Build history of the part. All positions in model axes, mm. Face numbers are marked on the shaded views. A direction names the side the tool comes from. Give positions to 0.01 mm unless a question says otherwise; leave off trailing zeros. Write each loop counter-clockwise with the first axis right and the second up, starting at its lowest first coordinate (ties: lowest second). Pieces come first, ordered by that corner, then holes.
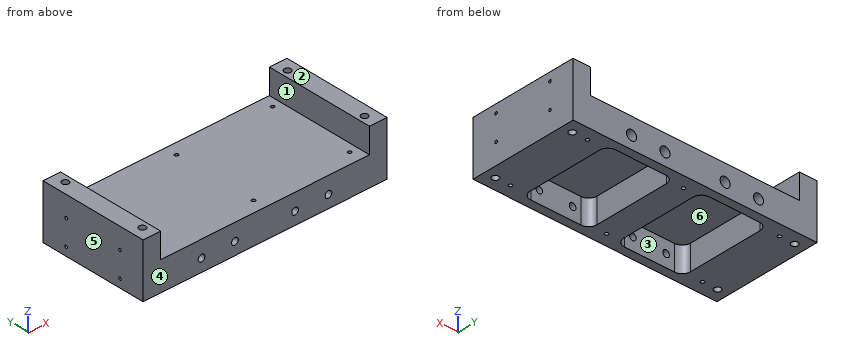
from build123d import *

# Parameters (mm, degrees)
SKETCH1_W                   = 292
SKETCH1_H                   = 35
BOSS_EXTRUDE1_DEPTH         = 130
SKETCH4_W                   = 21
SKETCH4_H                   = 130
BOSS_EXTRUDE2_DEPTH         = 30
SKETCH2_R                   = 4
CUT_EXTRUDE1_DEPTH          = 291.044824122
M5_TAPPED_HOLE1_D           = 4.2
TAP_DRILL_FOR_M4_TAP1_D     = 3.3
TAP_DRILL_FOR_M4_TAP1_DEPTH = 6
TAP_DRILL_FOR_M4_TAP1_TIP   = 0.991420021
TAP_DRILL_FOR_M4_TAP2_D     = 3.3
TAP_DRILL_FOR_M4_TAP2_DEPTH = 6
TAP_DRILL_FOR_M4_TAP2_TIP   = 0.991420021
CUT_EXTRUDE2_DEPTH          = 30
F_12_0MM_DOWEL_HOLE1_D      = 12
F_12_0MM_DOWEL_HOLE1_DEPTH  = 10
F_12_0MM_DOWEL_HOLE1_TIP    = 3.605163714
F_8_0MM_DOWEL_HOLE1_D       = 8
F_8_0MM_DOWEL_HOLE1_DEPTH   = 10
F_8_0MM_DOWEL_HOLE1_TIP     = 2.403442476


with BuildPart() as part:
    # Sketch1 → Boss-Extrude1 (new body)
    with BuildSketch(Plane(origin=(0, 0, 0), x_dir=(1, 0, 0), z_dir=(0, 1, 0))):
        with Locations((105, 47.5)):
            Rectangle(SKETCH1_W, SKETCH1_H)
    extrude(amount=BOSS_EXTRUDE1_DEPTH)

    # Sketch4 → Boss-Extrude2 (add)
    with BuildSketch(Plane.XY.offset(-30)):
        with Locations((-30.5, 65)):
            Rectangle(SKETCH4_W, SKETCH4_H)
        with Locations((240.5, 65)):
            Rectangle(SKETCH4_W, SKETCH4_H)
    extrude(amount=BOSS_EXTRUDE2_DEPTH)

    # Sketch2 → Cut-Extrude1 (cut, through all)
    with BuildSketch(Plane.XY.offset(-65)):
        with Locations(Location((238, 115, 0), (0, 0, 180))):
            Circle(SKETCH2_R)
        with Locations(Location((-28, 115, 0), (0, 0, 180))):
            Circle(SKETCH2_R)
        with Locations(Location((-28, 15, 0), (0, 0, 180))):
            Circle(SKETCH2_R)
        with Locations(Location((238, 15, 0), (0, 0, 180))):
            Circle(SKETCH2_R)
    extrude(amount=CUT_EXTRUDE1_DEPTH, mode=Mode.SUBTRACT)

    # M5 Tapped Hole1 (through all)
    with Locations(Plane.XY.offset(-30)):
        with Locations((-10, 115), (105, 115), (220, 115), (220, 15), (105, 15), (-10, 15)):
            Hole(M5_TAPPED_HOLE1_D / 2)

    # Tap Drill for M4 Tap1
    with Locations(Plane.ZY.offset(41)):
        with Locations((-55, 100), (-25, 100), (-55, 30), (-25, 30)):
            Hole(TAP_DRILL_FOR_M4_TAP1_D / 2, depth=TAP_DRILL_FOR_M4_TAP1_DEPTH)
            with Locations((0, 0, -(TAP_DRILL_FOR_M4_TAP1_DEPTH + TAP_DRILL_FOR_M4_TAP1_TIP / 2))):  # 118° drill point
                Cone(0, TAP_DRILL_FOR_M4_TAP1_D / 2, TAP_DRILL_FOR_M4_TAP1_TIP, mode=Mode.SUBTRACT)

    # Tap Drill for M4 Tap2
    with Locations(Plane(origin=(251, 0, 0), x_dir=(0, 0, -1), z_dir=(1, 0, 0))):
        with Locations((10, 100), (40, 100), (10, 30), (40, 30)):
            Hole(TAP_DRILL_FOR_M4_TAP2_D / 2, depth=TAP_DRILL_FOR_M4_TAP2_DEPTH)
            with Locations((0, 0, -(TAP_DRILL_FOR_M4_TAP2_DEPTH + TAP_DRILL_FOR_M4_TAP2_TIP / 2))):  # 118° drill point
                Cone(0, TAP_DRILL_FOR_M4_TAP2_D / 2, TAP_DRILL_FOR_M4_TAP2_TIP, mode=Mode.SUBTRACT)

    # Sketch31 → Cut-Extrude2 (cut)
    with BuildSketch(Plane(origin=(0, 0, -65), x_dir=(-1, 0, 0), z_dir=(0, 0, -1))):
        with BuildLine():
            Line((-191, 120), (-131, 120))
            ThreePointArc((-131, 120), (-123.928932188, 117.071067812), (-121, 110))
            Line((-121, 110), (-121, 20))
            ThreePointArc((-121, 20), (-123.928932188, 12.928932188), (-131, 10))
            Line((-131, 10), (-191, 10))
            ThreePointArc((-191, 10), (-198.071067812, 12.928932188), (-201, 20))
            Line((-201, 20), (-201, 110))
            ThreePointArc((-201, 110), (-198.071067812, 117.071067812), (-191, 120))
        make_face()
        with BuildLine():
            Line((-79, 120), (-19, 120))
            ThreePointArc((-19, 120), (-11.928932188, 117.071067812), (-9, 110))
            Line((-9, 110), (-9, 20))
            ThreePointArc((-9, 20), (-11.928932188, 12.928932188), (-19, 10))
            Line((-19, 10), (-79, 10))
            ThreePointArc((-79, 10), (-86.071067812, 12.928932188), (-89, 20))
            Line((-89, 20), (-89, 110))
            ThreePointArc((-89, 110), (-86.071067812, 117.071067812), (-79, 120))
        make_face()
    extrude(amount=-CUT_EXTRUDE2_DEPTH, mode=Mode.SUBTRACT)

    # Ø12.0mm Dowel Hole1
    with Locations(Plane(origin=(0, 130, 0), x_dir=(1, 0, 0), z_dir=(0, 1, 0))):
        with Locations((29, 50), (69, 50), (141, 50), (181, 50)):
            Hole(F_12_0MM_DOWEL_HOLE1_D / 2, depth=F_12_0MM_DOWEL_HOLE1_DEPTH)
            with Locations((0, 0, -(F_12_0MM_DOWEL_HOLE1_DEPTH + F_12_0MM_DOWEL_HOLE1_TIP / 2))):  # 118° drill point
                Cone(0, F_12_0MM_DOWEL_HOLE1_D / 2, F_12_0MM_DOWEL_HOLE1_TIP, mode=Mode.SUBTRACT)

    # Ø8.0mm Dowel Hole1
    with Locations(Plane(origin=(0, 10, 0), x_dir=(1, 0, 0), z_dir=(0, 1, 0))):
        with Locations((69, 50), (29, 50), (141, 50), (181, 50)):
            Hole(F_8_0MM_DOWEL_HOLE1_D / 2, depth=F_8_0MM_DOWEL_HOLE1_DEPTH)
            with Locations((0, 0, -(F_8_0MM_DOWEL_HOLE1_DEPTH + F_8_0MM_DOWEL_HOLE1_TIP / 2))):  # 118° drill point
                Cone(0, F_8_0MM_DOWEL_HOLE1_D / 2, F_8_0MM_DOWEL_HOLE1_TIP, mode=Mode.SUBTRACT)


solid = part.part
1. 3-axis set-ups, long thin cutter, end or side, ignore diameter. For the marked faces 1, 2 and 3: which of +Z, -Z, +X, -X, +Y, -Y reach the whole face in a straight line?
2. Saw through at A-A on x = 181. Give the cut face in (y, z).
3. Drop flat-ended pins along their axis: pin 1 (5 mm diameter, centred on x = 220, y = 115, fed in from +Z); pin 2 (24 mm diameter, centred on x = 170, z = -45.5, fed in from -Y); pin 3 (3 mm diameter, centred on x = 16, y = 101, fed in from -Z); pin 4 (9 mm diameter, centred on x = 69, z = -50, fed in from +Y). Give the stop position or say it passes through.
4. Saw through at C-C on x = 238. Give the cut face in (y, z), plus the area to 3 significant figures.
5. Drill centre lines: line 1 along Z through (x, y) = (246, 100); line 2 along Z through (x, y) = (-39, 30); line 3 along X through (y, z) = (91.5, -57). Where is each one in solid material? Low to high.
6. Saw through at B-B on y = 90. Give the cut face in (x, z).
7. Mould opens along X. For the marked faces 4, 5 and 6 say: pulls with the +X half, pulls with the -X half, needs draft (parallel to the pull), parting line crosses it, or undercut.
8. Saw through at D-D on x = 93. Give the cut face in (y, z).
Outcome:
1. face 1: +Z, +Y, -Y
1. face 2: +Z, +X, -X, +Y, -Y
1. face 3: -Z
2. outline: (0, -65) - (10, -65) - (10, -54) - (0, -54) - close; (0, -46) - (10, -46) - (10, -35) - (120, -35) - (120, -44) - (130, -44) - (130, -30) - (0, -30) - close; (120, -65) - (130, -65) - (130, -56) - (120, -56) - close
3. pin 1: stops at z = -30
3. pin 2: stops at y = 0
3. pin 3: stops at z = -35
3. pin 4: stops at y = 10
4. outline: (0, -65) - (11, -65) - (11, 0) - (0, 0) - close; (19, -65) - (111, -65) - (111, 0) - (19, 0) - close; (119, -65) - (130, -65) - (130, 0) - (119, 0) - close
4. area: 7,410 mm2
5. line 1: z = -65 to -41.65, -38.35 to -11.65, -8.35 to 0
5. line 2: z = -65 to -56.65, -53.35 to -26.65, -23.35 to 0
5. line 3: x = -41 to 9, 89 to 121, 201 to 251
6. outline: (-41, -65) - (9, -65) - (9, -35) - (89, -35) - (89, -65) - (121, -65) - (121, -35) - (201, -35) - (201, -65) - (251, -65) - (251, 0) - (230, 0) - (230, -30) - (-20, -30) - (-20, 0) - (-41, 0) - close
7. face 4: needs draft
7. face 5: pulls with the -X half
7. face 6: undercut
8. outline: (0, -65) - (130, -65) - (130, -30) - (0, -30) - close
